Verification items for the finished model (mm, model axes). A direction names the side the tool comes from. Round coordinates to 2 decimals unless told otherwise and drop trailing zeros. Loops run counter-clockwise (first coordinate to the right, second up) from the corner with the lowest first, then second, coordinate; pieces in that order, holes last. Notation, with made-up numbers: M 85.5,-16.75 L 95.5,-16.75 A23 ccw 95.5,3.25 Z; hole C 66.25,50 d8. An arc over 180 degrees is marked long. One line per item, written item: value.
from build123d import *

# Parameters (mm, degrees)
F0_W          = 30
F0_H          = 30
F1_DEPTH      = 50
F1_DEPTH_BACK = 50
F2_R          = 3
F3_T          = -1.5
F5_DEPTH      = 100.001


with BuildPart() as f1:
    # F0 (on Front) → F1 (new body, two sides)
    with BuildSketch(Plane.XZ) as f1_sk:
        Rectangle(F0_W, F0_H)
    extrude(amount=F1_DEPTH)
    extrude(f1_sk.sketch, amount=-F1_DEPTH_BACK)

    # F2
    f2_edges = [f1.edges().sort_by_distance(p)[0] for p in [
        (0, -50, 15),
        (0, 50, 15),
        (15, 0, 15),
        (15, -50, 0),
        (15, 50, 0),
    ]]
    fillet(f2_edges, radius=F2_R)

    # F3
    f3_openings = [f1.faces().sort_by_distance(p)[0] for p in [
        (-15, 0, -0.018475),
        (-0.018475, 0, -15),
    ]]
    offset(amount=F3_T, openings=f3_openings)

    # F4 (on face) → F5 (cut, through all)
    with BuildSketch(Plane.XZ.offset(50)):
        with BuildLine():
            Line((-15, -4.424621), (-9.712311, -9.712311))
            ThreePointArc((-9.712311, -9.712311), (-2.287689, -9.712311), (-2.287689, -2.287689))
            Line((-2.287689, -2.287689), (-15, 10.424621))
            Line((-15, 10.424621), (-15, -4.424621))
        make_face()
    extrude(amount=-F5_DEPTH, mode=Mode.SUBTRACT)


solid = f1.part
(1) Mould release check, pull along Y, two halves, no side actions. Record for faces 1 (the face through (-8.555, -49.26, 3.979)), 2 (the face through (1, 48.5, -1)), 3 (the face through (14.14, 49.1, -1.31)): +Y half, -Y half, draft (parallel to the pull), parting line (faces both ways), or undercut.
Completed:
face 1: draft
face 2: undercut
face 3: +Y half
(2) Sectioned sample at C-C on y = 29.5. Enter the section's corners in (x, z).
Completed:
outline: M -15,13.5 L 12,13.5 A1.5 cw 13.5,12 L 13.5,-15 L 15,-15 L 15,12 A3 ccw 12,15 L -15,15 Z
(3) Sectioned sample at D-D on x = 5.25. Enter the section's corners in (y, z), and give its area (3 significant figures).
Completed:
outline: M -50,-15 L -48.5,-15 L -48.5,12 A1.5 cw -47,13.5 L 47,13.5 A1.5 cw 48.5,12 L 48.5,-15 L 50,-15 L 50,12 A3 ccw 47,15 L -47,15 A3 ccw -50,12 Z
area: 233 mm^2
(4) Tool access check on faces 4 (the face through (1, -48.5, -1)), 5 (the face through (14, 0, -15)), 6 (the face through (-2, -1, 15)), 7 (the face through (-8.555, 49.24, 3.979)), 8 (the face through (-12.393, -49.26, -7.031)). Record the directions out of +Z, -Z, +X, -X, +Y, -Y that give a thin tool (end or side, any length) a straight path to the whole face; none if there is none.
Completed:
face 4: -Z, -X
face 5: -Z, +X, -X, +Y, -Y
face 6: +Z, +X, -X, +Y, -Y
face 7: -X, +Y, -Y
face 8: +Y, -Y
(5) Sectioned sample at A-A on z = -6. Enter the section's corners in (x, y).
Completed:
outline: M -15,-50 L -13.42,-50 L -13.42,-48.5 L -15,-48.5 Z; M -15,48.5 L -13.42,48.5 L -13.42,50 L -15,50 Z; M -0.75,-50 L 12,-50 A3 ccw 15,-47 L 15,47 A3 ccw 12,50 L -0.75,50 L -0.75,48.5 L 12,48.5 A1.5 cw 13.5,47 L 13.5,-47 A1.5 cw 12,-48.5 L -0.75,-48.5 Z
(6) Sectioned sample at B-B on x = -6. Enter the section's corners in (y, z).
Completed:
outline: M -50,-15 L -48.5,-15 L -48.5,-11.25 L -50,-11.25 Z; M -50,1.42 L -48.5,1.42 L -48.5,12 A1.5 cw -47,13.5 L 47,13.5 A1.5 cw 48.5,12 L 48.5,1.42 L 50,1.42 L 50,12 A3 ccw 47,15 L -47,15 A3 ccw -50,12 Z; M 48.5,-15 L 50,-15 L 50,-11.25 L 48.5,-11.25 Z
(7) Depth check by flat-ended pin: pin 1 Ø8 at (x, y) = (-2.5, 30) entering from -Z; pin 2 Ø10 at (y, z) = (-5.5, -12) entering from -X. Enter the tip coordinate at first touch or a pass-through.
Completed:
pin 1: stops at z = 13.5
pin 2: stops at x = 13.5
(8) Thickness scan on L1, parallel to Y at x = -0.5, z = -4.5; L2, parallel to X at y = 22.5, z = -13.25. Record the ranges inside material, lowest first. Write a range as from..to.
Completed:
L1: y = -50..-48.5, 48.5..50
L2: x = 13.5..15
